Design review of the part built by this model. Coordinates are the model's own, in mm. Coordinates: 2 decimals unless noted, no trailing zeros. Loops run counter-clockwise (first coordinate to the right, second up) from the corner with the lowest first, then second, coordinate; pieces in that order, holes last. Notation, with made-up numbers: (-32, -34) -> (27, -34) arc R26 cw to (27, -15) -> close; hole circle Ø3 at (46, 17.5). An arc over 180 degrees is marked (long way). Use a Markdown table: item, result. Add a question column.
Q1. Take a section at A-A on y = 0. Write out the cut boundary in (x, z).
Q2. Take a section at C-C on z = 3.55. Count the separate pieces of the cut face and the enclosed holes in it, plus the area to 3 significant figures.
Q3. For probe 1 along Y at (x, z) = (33, 4.75); probe 2 along X at (y, z) = (4.5, 1.3); probe 3 along X at (y, z) = (-14, 3.3), list the stretches that pass through material, from the lowest coordinate up.
Q4. Take a section at B-B on x = 172. Write out the cut boundary in (y, z), plus the area to 3 significant figures.
Q5. Clearance check with flat-ended pins moving along their axes: pin 1 Ø1 at (y, z) = (-12, 0.5) entering from +X; pin 2 Ø2.5 at (y, z) = (-9.5, 2) entering from +X; pin 3 Ø3.5 at (x, y) = (62.88, 8.45) entering from -Z; pin 4 Ø3 at (y, z) = (-9, 3.5) entering from +X. State where each tip first meets the part, or that it passes through.
from build123d import *

# Parameters (mm, degrees)
BOSS_EXTRUDE1_DEPTH = 5
SKETCH2_R           = 2
SKETCH2_R_2         = 1.979542606
CUT_EXTRUDE1_DEPTH  = 10
SKETCH3_R           = 2
CUT_EXTRUDE2_DEPTH  = 10


with BuildPart() as part:
    # Sketch1 → Boss-Extrude1 (new body)
    with BuildSketch(Plane.XY):
        with BuildLine():
            Line((0, 20), (200, 20))
            ThreePointArc((200, 20), (220, 0), (200, -20))
            Line((200, -20), (0, -20))
            ThreePointArc((0, -20), (-20, 0), (0, 20))
        make_face()
        Polygon((-0.621565279, -5), (-0.621565279, -15.35), (59.378434721, -15.35), (59.378434721, 15.35), (-0.621565279, 15.35), (-0.621565279, 5), (-3.621565279, 5), (-3.621565279, -5), align=None, mode=Mode.SUBTRACT)
        Polygon((140.672709247, -5), (140.672709247, -15.35), (200.672709247, -15.35), (200.672709247, 15.35), (140.672709247, 15.35), (140.672709247, 5), (137.672709247, 5), (137.672709247, -5), align=None, mode=Mode.SUBTRACT)
    extrude(amount=BOSS_EXTRUDE1_DEPTH)

    # Sketch2 → Cut-Extrude1 (cut)
    with BuildSketch(Plane(origin=(0, 0, 0), x_dir=(-1, 0, 0), z_dir=(0, 0, -1))):
        with Locations((-137.172709247, 8.45)):
            Circle(SKETCH2_R)
        with Locations((-137.172709247, -8.45)):
            Circle(SKETCH2_R_2)
        with Locations((-204.172709247, 8.45)):
            Circle(SKETCH2_R)
        with Locations((-204.172709247, -8.45)):
            Circle(SKETCH2_R)
    extrude(amount=-CUT_EXTRUDE1_DEPTH, mode=Mode.SUBTRACT)

    # Sketch3 → Cut-Extrude2 (cut)
    with BuildSketch(Plane(origin=(0, 0, 0), x_dir=(-1, 0, 0), z_dir=(0, 0, -1))):
        with Locations((4.121565279, 8.45)):
            Circle(SKETCH3_R)
        with Locations((4.121565279, -8.45)):
            Circle(SKETCH3_R)
        with Locations((-62.878434721, -8.45)):
            Circle(SKETCH3_R)
        with Locations((-62.878434721, 8.45)):
            Circle(SKETCH3_R)
    extrude(amount=-CUT_EXTRUDE2_DEPTH, mode=Mode.SUBTRACT)


solid = part.part
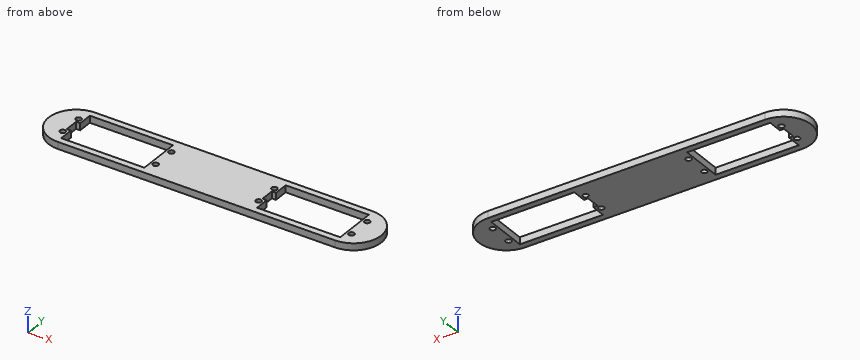
Answer list:
| question | item | result |
|---|---|---|
| 1 | outline | (-20, 0) -> (-3.62, 0) -> (-3.62, 5) -> (-20, 5) -> close; (59.38, 0) -> (137.67, 0) -> (137.67, 5) -> (59.38, 5) -> close; (200.67, 0) -> (220, 0) -> (220, 5) -> (200.67, 5) -> close |
| 2 | separate pieces | 1 |
| 2 | enclosed holes | 10 |
| 2 | area | 5,410 mm² |
| 3 | probe 1 | -20 to -15.35, 15.35 to 20 |
| 3 | probe 2 | -19.49 to -3.62, 59.38 to 137.67, 200.67 to 219.49 |
| 3 | probe 3 | -14.28 to -0.62, 59.38 to 140.67, 200.67 to 214.28 |
| 4 | outline | (-20, 0) -> (-15.35, 0) -> (-15.35, 5) -> (-20, 5) -> close; (15.35, 0) -> (20, 0) -> (20, 5) -> (15.35, 5) -> close |
| 4 | area | 46.5 mm² |
| 5 | pin 1 | x = 216.36 |
| 5 | pin 2 | x = 218.22 |
| 5 | pin 3 | through |
| 5 | pin 4 | x = 218.54 |
